Here's how the part is built. I have some questions about the finished solid (model axes, mm). A direction names the side the tool comes from. Round coordinates to 2 decimals unless told otherwise and drop trailing zeros. Write each loop counter-clockwise with the first axis right and the second up, starting at its lowest first coordinate (ties: lowest second). Pieces come first, ordered by that corner, then holes. Notation, with made-up numbers: (-30, 63) -> (17, 63) arc R9 cw to (17, 79) -> close; hole circle Ø7 at (3.25, 1.25). An arc over 180 degrees is marked (long way). Put each result on its own line as item: value. Start each with the question number.
1. Which directions (+Z, -Z, +X, -X, +Y, -Y) give clear straight access to the entire face, cutting with the end or side of a thin tool? Please do faces 4 (the face through (-75.059, 1.958, 18.226)), 5 (the face through (-12, 0, -30)).
2. I need wall thicknesses on probe 1 along Z at (x, y) = (-30, -2.2); probe 2 along Z at (x, y) = (-70, 0.35); probe 3 along Z at (x, y) = (-6, 0). Which ranges of each line are inside material? Lowest first, please. Write a range as from..to.
3. Suppose I cut it at D-D (z = 14). Count the separate pieces of the cut face and the enclosed holes in it, then the cut area to 3 significant figures.
4. Suppose I cut it at C-C (x = -6). Please give me the cut outline in (y, z).
5. For pin 1 (11 mm diameter, centred on x = -70, z = -15, fed in from +Y), with a flat end and sliding along its axis, tell me the tip position at first contact or that it passes through.
6. We'd pull the mould along X, two halves only. Please class faces 1 (the face through (-25, -5, 0)), 2 (the face through (-80, 0, 0)), 3 (the face through (-67, -1, -12)): +X half, -X half, draft (parallel to the pull), parting line (faces both ways), or undercut.
7. Suppose I cut it at A-A (x = -50). Please give me the cut outline in (y, z), then the cut area to 3 significant figures.
8. Suppose I cut it at B-B (z = 0). Please give me the cut outline in (x, y).
Autodesk Inventor part; units mm, degrees
ref_plane "YZ Plane" through (0, 0, 0) normal (1, 0, 0) x (0, 1, 0)
ref_plane "XZ Plane" through (0, 0, 0) normal (0, 1, 0) x (-1, 0, 0)
ref_plane "XY Plane" through (0, 0, 0) normal (0, 0, 1) x (1, 0, 0)
sketch "Sketch6" plane through (0, -5, 0) normal (0, -1, 0) x (1, 0, 0)
  circle A0 centre (-30, 15) radius 3.25
  circle A1 centre (-30, -15) radius 3.25
  circle A2 centre (-50, -15) radius 3.25
  circle A3 centre (-50, 15) radius 3.25
  circle A4 centre (-70, 15) radius 3.25
  circle A5 centre (-70, -15) radius 3.25
  point P0 (0, 0)
sketch "Sketch1" plane through (0, 0, 0) normal (0, 1, 0) x (-1, 0, 0)
  line L0 (-98, 30) -> (98, 30)
  line L1 (100, 28) -> (100, -28)
  line L2 (98, -30) -> (-98, -30)
  line L3 (-100, -28) -> (-100, 28)
  line L4 (-100, 30) -> (100, -30) construction
  line L5 (100, 30) -> (-100, -30) construction
  arc A0 (-98, 30) -> (-100, 28) centre (-98, 28) ccw
  arc A1 (100, 28) -> (98, 30) centre (98, 28) ccw
  arc A2 (98, -30) -> (100, -28) centre (98, -28) ccw
  arc A3 (-100, -28) -> (-98, -30) centre (-98, -28) ccw
  circle A4 centre (-22, 0) radius 22
  circle A5 centre (-50, 0) radius 3.75
  circle A6 centre (6, 0) radius 3.75
  circle A7 centre (30, 15) radius 3.25
  circle A8 centre (50, 15) radius 3.25
  circle A9 centre (70, 15) radius 3.25
  circle A10 centre (30, -15) radius 3.25
  circle A11 centre (50, -15) radius 3.25
  circle A12 centre (70, -15) radius 3.25
  point P0 (0, 0)
  point P1 (-100, 0)
  dimension "d0" = 60
  dimension "d1" = 200
  dimension "d2" = 2
  dimension "d3" = 44
  dimension "d4" = 56
  dimension "d5" = 28
  dimension "d6" = 7.5
  dimension "d7" = 7.5
  dimension "d8" = 50
  dimension "d9" = 6.5
  dimension "d10" = 6.5
  dimension "d11" = 6.5
  dimension "d12" = 6.5
  dimension "d13" = 6.5
  dimension "d14" = 6.5
  dimension "d15" = 15
  dimension "d16" = 30
  dimension "d17" = 30
  dimension "d18" = 20
  dimension "d19" = 20
extrude "Plate1" add sketch "Sketch1" along normal mid plane 10 contours L0 A1 L1 A2 L2 A3 L3 A0 | A7 | A8 | A9 | A10 | A11 | A12
sketch "Sketch2" plane through (0, 5, 0) normal (0, 1, 0) x (1, 0, 0)
  line L0 (98, -30) -> (-98, -30)
  line L1 (100, 30) -> (60, 30)
  line L2 (60, 30) -> (60, -30)
  line L3 (60, -30) -> (100, -30)
  line L4 (100, -30) -> (100, 30)
  line L5 (100, 28) -> (100, -28)
  line L6 (-98, 30) -> (98, 30)
  point P0 (0, 0)
  dimension "d21" = 40
extrude "Cut1" cut sketch "Sketch2" against normal blind 10
fillet "Corner Round1" radius 2 2 edges at (60, 0, -30) (60, 0, 30)
sketch "Sketch3" plane through (0, 5, 0) normal (0, 1, 0) x (1, 0, 0)
  circle A0 centre (50, 0) radius 3.75
  circle A1 centre (-6, 0) radius 3.75
  point P0 (0, 0)
sketch "Sketch4" plane through (0, 5, 0) normal (0, 1, 0) x (1, 0, 0)
  line L0 (-100, -28) -> (-100, 28) construction
  line L1 (-98, 30) -> (58, 30) construction
  line L2 (58, -30) -> (-98, -30)
  line L3 (-100, 30) -> (-80, 30)
  line L4 (-80, 30) -> (-80, -30)
  line L5 (-80, -30) -> (-100, -30)
  line L6 (-100, -30) -> (-100, 30)
  point P0 (0, 0)
  dimension "d25" = 20
extrude "Cut2" cut sketch "Sketch4" against normal blind 10
sketch "Sketch5" plane through (0, 5, 0) normal (0, 1, 0) x (1, 0, 0)
  point P0 (0, 0)
  point P1 (-30, -15)
  point P2 (-30, -15)
  point P3 (-50, -15)
  point P4 (-50, -15)
  point P5 (-70, -15)
  point P6 (-70, -15)
  point P7 (-70, 15)
  point P8 (-70, 15)
  point P9 (-50, 15)
  point P10 (-50, 15)
  point P11 (-30, 15)
  point P12 (-30, 15)
hole "Hole1" at (-70, 5, 15) at (-70, 5, -15) at (-50, 5, -15) at (-30, 5, -15) at (-30, 5, 15) at (-50, 5, 15) direction (0, -1, 0) diameter 7 end through all counterbore diameter 12 counterbore depth 6
equation "\"d7\" = d6"
equation "\"d10\" = d9"
equation "\"d11\" = d9"
equation "\"d12\" = d9"
equation "\"d13\" = d9"
equation "\"d14\" = d9"
equation "\"d22\" = Thickness"
equation "\"d26\" = Thickness"
equation "\"d20\" = Thickness"
equation "\"BendReliefDepth\" = 0.5 * Thickness"
properties part number "HCMUTE-CDT23-BAT_TRUC_DAN" material "Stainless Steel"
Verdict:
1. face 4: +Y
1. face 5: -Z, +X, -X, +Y, -Y
2. probe 1: z = -30..-18.5, -11.5..11.5, 18.5..30
2. probe 2: z = -30..-21, -9..9, 21..30
2. probe 3: z = -30..-3.75, 3.75..30
3. separate pieces: 5
3. enclosed holes: 0
3. area: 767 mm^2
4. outline: (-5, -30) -> (5, -30) -> (5, -3.75) -> (-5, -3.75) -> close; (-5, 3.75) -> (5, 3.75) -> (5, 30) -> (-5, 30) -> close
5. pin 1: stops at y = -1
6. face 1: draft
6. face 2: -X half
6. face 3: undercut
7. outline: (-5, -30) -> (5, -30) -> (5, -21) -> (-1, -21) -> (-1, -18.5) -> (-5, -18.5) -> close; (-5, -11.5) -> (-1, -11.5) -> (-1, -9) -> (5, -9) -> (5, 9) -> (-1, 9) -> (-1, 11.5) -> (-5, 11.5) -> close; (-5, 18.5) -> (-1, 18.5) -> (-1, 21) -> (5, 21) -> (5, 30) -> (-5, 30) -> close
7. area: 400 mm^2
8. outline: (-80, -5) -> (-9.75, -5) -> (-9.75, 5) -> (-80, 5) -> close; (-2.25, -5) -> (0, -5) -> (0, 5) -> (-2.25, 5) -> close; (44, -5) -> (46.25, -5) -> (46.25, 5) -> (44, 5) -> close; (53.75, -5) -> (60, -5) -> (60, 5) -> (53.75, 5) -> close
